Print and shaded views of the part. All mm, measured from the part's lowest x, y and z. A direction names the side the tool comes from. Round coordinates to 2 decimals unless told otherwise and drop trailing zeros. Write each loop counter-clockwise with the first axis right and the second up, starting at its lowest first coordinate (ties: lowest second). Pieces come first, ordered by that corner, then holes. Notation, with made-up numbers: (79.5, 7.5) - (88.5, 7.5) arc R20 ccw to (88.5, 43.5) - close; hole circle Ø4 at (-18.75, -35). An arc over 180 degrees is marked (long way). One line per item, written item: value.
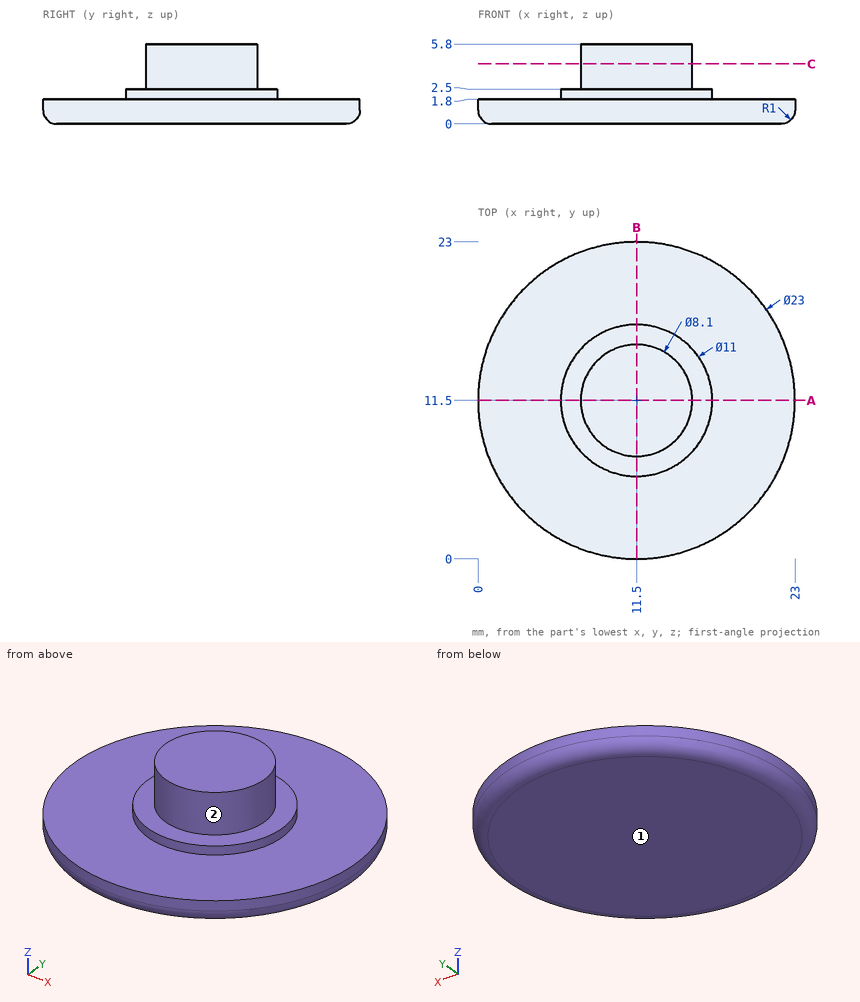
1. Band-saw the part on C-C on z = 4.35. Write the cut outline in (x, y).
Report:
outline: circle Ø8.1 at (11.5, 11.5)
2. Tool access for the marked faces 1 and 2: list every direction of +Z, -Z, +X, -X, +Y, -Y with a clear straight run to the whole face (end or side of a thin tool).
Report:
face 1: -Z, +X, -X, +Y, -Y
face 2: +Z
3. Wall check: probe 1 along Z at (x, y) = (3.5, 8.5); probe 2 along Z at (x, y) = (7.5, 13.5); probe 3 along X at (y, z) = (11, 4.55). Give the ranges that are in metal, low to high. Write a range as [from, to].
Report:
probe 1: [0, 1.8]
probe 2: [0, 2.5]
probe 3: [7.48, 15.52]
4. Band-saw the part on A-A on y = 11.5. Write the cut outline in (x, z).
Report:
outline: (0, 1) arc R1 ccw to (1, 0) - (22, 0) arc R1 ccw to (23, 1) - (23, 1.8) - (17, 1.8) - (17, 2.5) - (15.55, 2.5) - (15.55, 5.8) - (7.45, 5.8) - (7.45, 2.5) - (6, 2.5) - (6, 1.8) - (0, 1.8) - close
5. Drop flat-ended pins along their axis: pin 1 (1.5 mm diameter, centred on x = 19.5, z = 1.5, fed in from -Y); pin 2 (8 mm diameter, centred on x = 7.5, y = 16, fed in from -Z); pin 3 (2 mm diameter, centred on x = 19.5, y = 19, fed in from +Z). Give the stop position or say it passes through.
Report:
pin 1: y = 2.57
pin 2: z = 0
pin 3: z = 1.8
